from build123d import *

# Parameters (mm, degrees)
SKETCH5_W           = 44
SKETCH5_H           = 24
BOSS_EXTRUDE3_DEPTH = 15
SHELL1_T            = -2
SKETCH7_W           = 2
SKETCH7_H           = 11.017608059
BOSS_EXTRUDE4_DEPTH = 10
SKETCH9_W           = 150
SKETCH9_H           = 2
BOSS_EXTRUDE5_DEPTH = 20


with BuildPart() as part:
    # Sketch5 → Boss-Extrude3 (new body)
    with BuildSketch(Plane(origin=(0, 0, 0), x_dir=(1, 0, 0), z_dir=(0, 1, 0))):
        Rectangle(SKETCH5_W, SKETCH5_H)
    extrude(amount=BOSS_EXTRUDE3_DEPTH)

    # Shell1
    shell1_openings = [part.faces().sort_by_distance(p)[0] for p in [
        (0, 7.5, -12),
    ]]
    offset(amount=SHELL1_T, openings=shell1_openings, kind=Kind.INTERSECTION)

    # Sketch7 → Boss-Extrude4 (add)
    with BuildSketch(Plane(origin=(-20, 0, 0), x_dir=(0, 0, -1), z_dir=(1, 0, 0))):
        with Locations((11, 7.49119597)):
            Rectangle(SKETCH7_W, SKETCH7_H)
    boss_extrude4 = extrude(amount=BOSS_EXTRUDE4_DEPTH)

    # Mirror1: Boss-Extrude4 across plane
    add(boss_extrude4.mirror(Plane(origin=(0, 0, 0), x_dir=(0, 0, 1), z_dir=(1, 0, 0))))

    # Sketch9 → Boss-Extrude5 (add)
    with BuildSketch(Plane(origin=(0, 0, -12), x_dir=(-1, 0, 0), z_dir=(0, 0, -1))):
        with Locations((0, 1)):
            Rectangle(SKETCH9_W, SKETCH9_H)
    extrude(amount=BOSS_EXTRUDE5_DEPTH)


solid = part.part
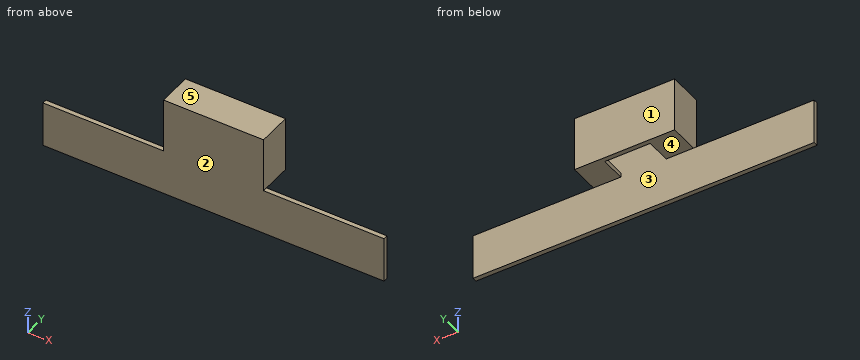
Read the model definition and answer for the solid it produces. Units are mm, in the model's axes. Face numbers are marked on the shaded views. A direction names the side the tool comes from. Round coordinates to 2 decimals unless told otherwise and drop trailing zeros. Write each loop counter-clockwise with the first axis right and the second up, starting at its lowest first coordinate (ties: lowest second). Pieces come first, ordered by that corner, then holes. Notation, with made-up numbers: (25.25, -20.75) - (60.25, -20.75) arc R8 ccw to (60.25, -7.75) - close; hole circle Ø1 at (-12, 14.25). An arc over 180 degrees is marked (long way). Use a Markdown table: item, result.
(1) The mould has two halves that part along Y. Classify the marked faces 1, 2 and 3: released by +Y, released by -Y, zero draft, split by the parting line, or undercut.
Reported:
| item | result |
|---|---|
| face 1 | released by +Y |
| face 2 | released by -Y |
| face 3 | undercut |
(2) The part is cut by section D-D (z = -23.5). Write down the section's boundary in (x, y), then the cut area to 3 significant figures.
Reported:
| item | result |
|---|---|
| outline | (-75, 0) - (75, 0) - (75, 2) - (-75, 2) - close |
| area | 300 mm2 |
(3) Which of the six approach directions +Z, -Z, +X, -X, +Y, -Y give full straight-line access (tool end or side, diameter ignored) to the marked faces 4 and 5?
Reported:
| item | result |
|---|---|
| face 4 | -Z, +X, -X, +Y |
| face 5 | +Z, +X, -X, +Y, -Y |
(4) Straight lines are drawn through the part: line 1 along Y through (x, z) = (13, 9); line 2 along X through (y, z) = (5.5, -2); line 3 along X through (y, z) = (8.25, -11.5). For each, find the intervals that lie inside material, in ascending order. Write a range as [from, to].
Reported:
| item | result |
|---|---|
| line 1 | [0, 2], [13, 15] |
| line 2 | [-22, -20], [20, 22] |
| line 3 | [-22, -10], [10, 22] |
(5) Each of these flat-tipped pins is pushed along its axis until it touches: pin 1 Ø2 at (x, y) = (58.5, 1) entering from +Z; pin 2 Ø5.5 at (y, z) = (10, 0.5) entering from -X; pin 3 Ø3 at (x, z) = (-53.5, -14.5) entering from +Y; pin 4 Ø11 at (x, z) = (-1, -1) entering from -Y. Where does it stop, or does it pass through?
Reported:
| item | result |
|---|---|
| pin 1 | z = -12 |
| pin 2 | x = -22 |
| pin 3 | y = 2 |
| pin 4 | y = 0 |
(6) The part is cut by section C-C (x = 53.5). Write down the section's boundary in (y, z), then the cut area to 3 significant figures.
Reported:
| item | result |
|---|---|
| outline | (0, -32) - (2, -32) - (2, -12) - (0, -12) - close |
| area | 40.0 mm2 |
(7) The part is cut by section A-A (z = 1.5). Write down the section's boundary in (x, y), then the cut area to 3 significant figures.
Reported:
| item | result |
|---|---|
| outline | (-22, 0) - (22, 0) - (22, 15) - (-22, 15) - close; hole (-20, 2) - (20, 2) - (20, 13) - (-20, 13) - close |
| area | 220 mm2 |
(8) The part is cut by section B-B (y = 10.5). Write down the section's boundary in (x, z), then the cut area to 3 significant figures.
Reported:
| item | result |
|---|---|
| outline | (-22, -12) - (-10, -12) - (-10, -10) - (-20, -10) - (-20, 10) - (20, 10) - (20, -10) - (10, -10) - (10, -12) - (22, -12) - (22, 12) - (-22, 12) - close |
| area | 216 mm2 |
